from build123d import *

# Parameters (mm, degrees)
BOSS_EXTRUDE1_DEPTH = 15
SKETCH4_R           = 1
BOSS_EXTRUDE3_DEPTH = 10
SKETCH5_R           = 1
BOSS_EXTRUDE4_DEPTH = 2.5
CUT_EXTRUDE1_REACH  = 43.608
SKETCH6_W           = 10
SKETCH6_H           = 5
FILLET1_R           = 7.5
FILLET2_R           = 5
SKETCH7_W           = 2
SKETCH7_H           = 4
BOSS_EXTRUDE5_DEPTH = 4
SKETCH8_R           = 1
BOSS_EXTRUDE6_DEPTH = 2


with BuildPart() as part:
    # Sketch1 → Boss-Extrude1 (new body)
    with BuildSketch(Plane(origin=(0, 0, 0), x_dir=(1, 0, 0), z_dir=(0, 1, 0))):
        Polygon((-7.5, -17.5), (-7.5, 20), (7.5, 20), (7.5, -17.5), (5, -17.5), (5, 17.5), (-5, 17.5), (-5, -17.5), align=None)
    extrude(amount=BOSS_EXTRUDE1_DEPTH)

    # Sketch4 → Boss-Extrude3 (add)
    with BuildSketch(Plane.ZY.offset(-5)):
        with Locations(Location((0, 7.5, 0), (0, 0, 180))):
            Circle(SKETCH4_R)
    extrude(amount=BOSS_EXTRUDE3_DEPTH)

    # Sketch5 → Boss-Extrude4 (add)
    with BuildSketch(Plane(origin=(7.5, 0, 0), x_dir=(0, 0, -1), z_dir=(1, 0, 0))):
        with Locations(Location((-12.5, 7.5, 0), (0, 0, 180))):
            Circle(SKETCH5_R)
    extrude(amount=BOSS_EXTRUDE4_DEPTH)

    # Sketch6 → Cut-Extrude1 (cut, up to next)
    with BuildSketch(Plane(origin=(0, 0, -20), x_dir=(-1, 0, 0), z_dir=(0, 0, -1)), mode=Mode.PRIVATE) as cut_extrude1_sk1:
        with Locations((0, 2.5)):
            Rectangle(SKETCH6_W, SKETCH6_H)
    cut_extrude1_tool1 = extrude(cut_extrude1_sk1.sketch, amount=-CUT_EXTRUDE1_REACH, mode=Mode.PRIVATE) & part.part
    add(cut_extrude1_tool1.solids().sort_by_distance((0, 2.5, -20))[0], mode=Mode.SUBTRACT)

    # Fillet1
    fillet1_edges = [part.edges().sort_by_distance(p)[0] for p in [
        (-6.25, 0, 17.5),
        (-6.25, 15, 17.5),
        (6.25, 0, 17.5),
        (6.25, 15, 17.5),
    ]]
    fillet(fillet1_edges, radius=FILLET1_R - 0.0001)  # a hair under: the kernel refuses the full size

    # Fillet2
    fillet2_edges = [part.edges().sort_by_distance(p)[0] for p in [
        (6.25, 0, -20),
        (-6.25, 0, -20),
    ]]
    fillet(fillet2_edges, radius=FILLET2_R)

    # Sketch7 → Boss-Extrude5 (add)
    with BuildSketch(Plane.XY.offset(-17.5)):
        with Locations((-1, 11)):
            Rectangle(SKETCH7_W, SKETCH7_H)
    extrude(amount=BOSS_EXTRUDE5_DEPTH)

    # Sketch8 → Boss-Extrude6 (add)
    with BuildSketch(Plane(origin=(0, 0, 0), x_dir=(0, 0, -1), z_dir=(1, 0, 0))):
        with Locations(Location((15.5, 11, 0), (0, 0, 270))):
            Circle(SKETCH8_R)
    extrude(amount=BOSS_EXTRUDE6_DEPTH)


solid = part.part
Input: part model. Units: mm. Frame: model coordinates. A direction names the side the tool comes from. Round coordinates to 2 decimals unless told otherwise and drop trailing zeros. Order: outer loops, then holes, each group sorted by start corner. A loop starts at its lowest first (then second) coordinate and runs counter-clockwise, first axis right, second up. Notation, with made-up numbers: (13, 62.25) - (58, 62.25) arc R18 cw to (58, 74.25) - close; hole circle Ø10 at (23.25, -20.75). An arc over 180 degrees is marked (long way). Answer as a JSON object with one key per item and string values. Group by question number.
(1) Cut plane B-B (z = -8). Return loops of the section in (x, y), then the cut area to 3 significant figures.
(2) Cut plane D-D (z = 0). Return loops of the section in (x, y), then the cut area to 3 significant figures.
(3) Draft query along X for faces 6 (the face through (6, 0, -3)), 7 (the face through (-2, 11, -16)), 8 (the face through (7.5, 7, -2)). Return one class per face: released by +X, released by -X, zero draft, split by the parting line, or undercut.
(4) Cut plane C-C (y = 3). Return loops of the section in (x, z), then the cut area to 3 significant figures.
(5) Reachability of faces 1 (the face through (0, 10, -20)), 2 (the face through (6, 2, -19)), 3 (the face through (2, 11, -16)), 4 (the face through (8.732, 6.824, 11.763)), 5 (the face through (0.07, 6.51, 0.13)) from +Z, -Z, +X, -X, +Y, -Y: full face, straight path, thin tool, end or side. Return the list, or none.
(6) Material intervals for probe 1 along X at (y, z) = (6.5, -4); probe 2 along Z at (x, y) = (3.5, 14); probe 3 along Z at (x, y) = (5.25, 8.25), sorted ascending. Write a range as from..to.
(7) Cut plane A-A (x = -0.5). Return loops of the section in (y, z), then the cut area to 3 significant figures.
(8) Pin query (flat end, axial travel): P1, Ø1, axis at x = -1.5, z = -15.5, coming from the -Y side; P2, Ø4.5, axis at y = 8.5, z = 1, coming from the +X side; P3, Ø3, axis at x = 0, z = -19, coming from the -Y side. Return the tip coordinate at first contact, or that it passes through.
Here are the results:
{
 "1": {"outline": "(-7.5, 0) - (-5, 0) - (-5, 15) - (-7.5, 15) - close; (5, 0) - (7.5, 0) - (7.5, 15) - (5, 15) - close", "area": "75.0 mm^2"},
 "2": {"outline": "(-7.5, 0) - (-5, 0) - (-5, 6.5) - (5, 6.5) - (5, 0) - (7.5, 0) - (7.5, 15) - (5, 15) - (5, 8.5) - (-5, 8.5) - (-5, 15) - (-7.5, 15) - close", "area": "95.0 mm^2"},
 "3": {"face 6": "zero draft", "face 7": "undercut", "face 8": "released by +X"},
 "4": {"outline": "(-7.5, -19.58) - (-5, -19.58) - (-5, 16) - (-7.5, 16) - close; (5, -19.58) - (7.5, -19.58) - (7.5, 16) - (5, 16) - close", "area": "178 mm^2"},
 "5": {"face 1": "-Z, +X, -X, +Y, -Y", "face 2": "-Z, +X, -X, -Y", "face 3": "+Z, +Y, -Y", "face 4": "+X", "face 5": "none"},
 "6": {"probe 1": "x = -7.5..-5, 5..7.5", "probe 2": "z = -20..-17.5", "probe 3": "z = -20..17.46"},
 "7": {"outline": "(5, -20) - (15, -20) - (15, -17.5) - (13, -17.5) - (13, -13.5) - (9, -13.5) - (9, -17.5) - (5, -17.5) - close; circle Ø2 at (7.5, 0)", "area": "44.1 mm^2"},
 "8": {"P1": "stops at y = 9", "P2": "stops at x = 7.5", "P3": "stops at y = 5"}
}
